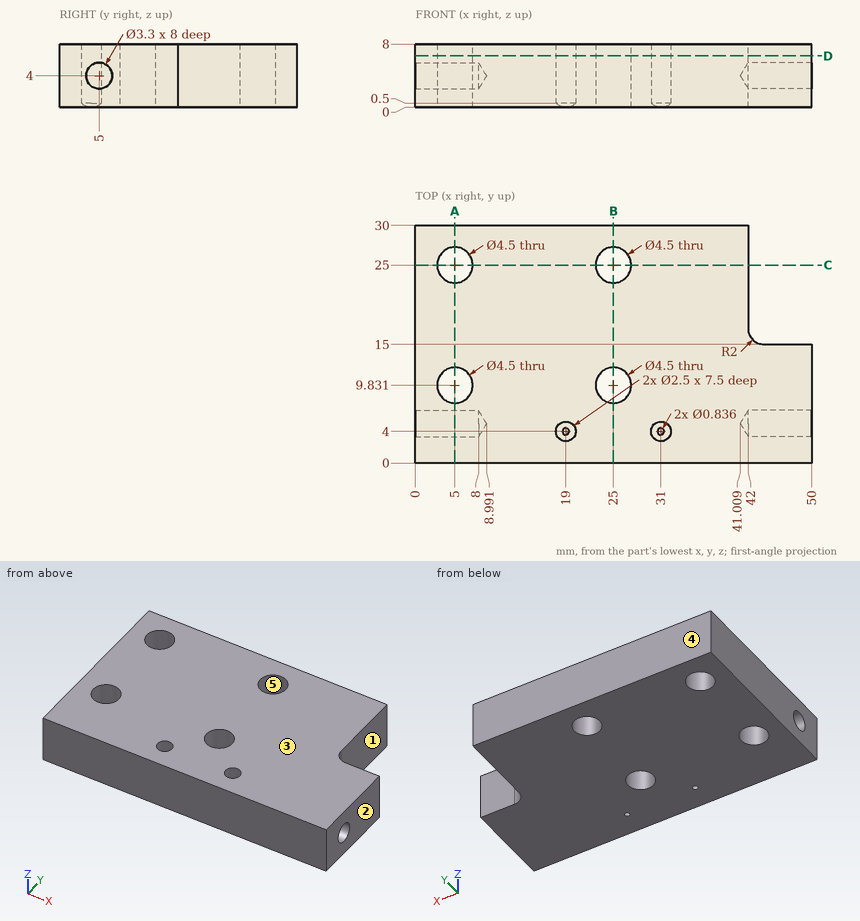
Design review of the part shown in the three views and the two pictorial views. Dimensions are in mm from the part's minimum x, y and z. A direction names the side the tool comes from. Coordinates: 2 decimals unless noted, no trailing zeros. Loops run counter-clockwise (first coordinate to the right, second up) from the corner with the lowest first, then second, coordinate; pieces in that order, holes last.
Q1. We need section D-D on z = 6.5. State the section outline as (x, y) points, and give its area (3 significant figures).
Reported:
outline: (0, 0) - (50, 0) - (50, 15) - (44, 15) arc R2 cw to (42, 17) - (42, 30) - (0, 30) - close; hole circle Ø4.5 at (5, 9.83); hole circle Ø4.5 at (5, 25); hole circle Ø2.5 at (19, 4); hole circle Ø4.5 at (25, 9.83); hole circle Ø4.5 at (25, 25); hole circle Ø2.5 at (31, 4)
area: 1,310 mm2
Q2. We need section B-B on x = 25. State the section outline as (y, z) points, and give its area (3 significant figures).
Reported:
outline: (0, 0) - (7.58, 0) - (7.58, 8) - (0, 8) - close; (12.08, 0) - (22.75, 0) - (22.75, 8) - (12.08, 8) - close; (27.25, 0) - (30, 0) - (30, 8) - (27.25, 8) - close
area: 168 mm2
Q3. We need section C-C on y = 25. State the section outline as (x, z) points.
Reported:
outline: (0, 0) - (2.75, 0) - (2.75, 8) - (0, 8) - close; (7.25, 0) - (22.75, 0) - (22.75, 8) - (7.25, 8) - close; (27.25, 0) - (42, 0) - (42, 8) - (27.25, 8) - close
Q4. Tool access review of the marked faces 1 and 2: name each direction out of +Z, -Z, +X, -X, +Y, -Y from which nothing blocks a thin tool from reaching the whole face with its end or side.
Reported:
face 1: +Z, -Z, +X, +Y
face 2: +Z, -Z, +X, +Y, -Y
Q5. To check wall thickness, follow line 1 (Y direction, x = 5, z = 2); line 2 (X direction, y = 10, z = 7); line 3 (X direction, y = 23, z = 1.5) (1 decimal). State the ranges of each line that lie inside material, in increasing order.
Reported:
line 1: y = 0 to 7.58, 12.08 to 22.75, 27.25 to 30
line 2: x = 0 to 2.76, 7.24 to 22.76, 27.24 to 50
line 3: x = 0 to 4, 6 to 24, 26 to 42
Q6. For pin 1 (2.5 mm diameter, centred on x = 5, y = 9.83, fed in from +Z); pin 2 (2 mm diameter, centred on x = 31, y = 4, fed in from +Z); pin 3 (2 mm diameter, centred on y = 5, z = 4, fed in from +X), all flat-tipped, find the tip position at first contact; note any pin that passes through.
Reported:
pin 1: passes through
pin 2: stops at z = 0.35
pin 3: stops at x = 41.61
Q7. The part is to be moulded in two halves that separate along Y. For the marked faces 3, 4 and 5, say which applies: +Y half, -Y half, draft (parallel to the pull), parting line (faces both ways), or undercut.
Reported:
face 3: draft
face 4: +Y half
face 5: undercut
Q8. We need section A-A on x = 5. State the section outline as (y, z) points.
Reported:
outline: (0, 0) - (7.58, 0) - (7.58, 8) - (0, 8) - close; (12.08, 0) - (22.75, 0) - (22.75, 8) - (12.08, 8) - close; (27.25, 0) - (30, 0) - (30, 8) - (27.25, 8) - close; hole circle Ø3.3 at (5, 4)
